Job drawing, mm, ordinate dimensions from the low corner. One solid piece. A direction names the side the tool comes from. Give positions to 0.01 mm unless a question says otherwise; leave off trailing zeros. Order: outer loops, then holes, each group sorted by start corner. A loop starts at its lowest first (then second) coordinate and runs counter-clockwise, first axis right, second up. Notation, with made-up numbers: M -1,75.5 L 12,75.5 A17 ccw 12,80.5 Z; hole C 48,87.5 d9. An arc over 180 degrees is marked long. Use CSV: the item, a comma, the result in double quotes. Start each with the question number.
Item 1: Band-saw the part on B-B on z = 31. Write the cut outline in (x, y).
Item 2: Band-saw the part on C-C on y = 132. Write the cut outline in (x, z).
Item 3: Wall check: line 1 along Z through (x, y) = (9, 16.25); line 2 along Y through (x, z) = (26, 17); line 3 along X through (y, z) = (132.5, 51). Give the ranges that are in metal, low to high.
Item 4: Pin check, flat tips, straight feed: P1, Ø6, axis at x = 108, y = 113, coming from the +Z side; P2, Ø9, axis at x = 6.5, y = 79, coming from the +Z side; P3, Ø4, axis at x = 21, y = 108, coming from the +Z side. Stop position of each tip, or through.
Item 5: Which spindle directions (+Z, -Z, +X, -X, +Y, -Y) get a long thin tool onto all of the face, cutting with end or side? Do the marked faces 1, 2 and 3. Say none if no direction does.
Item 6: Band-saw the part on A-A on x = 45.5. Write the cut outline in (y, z), plus the area to 3 significant figures.
Item 7: Band-saw the part on D-D on x = 9. Write the cut outline in (y, z).
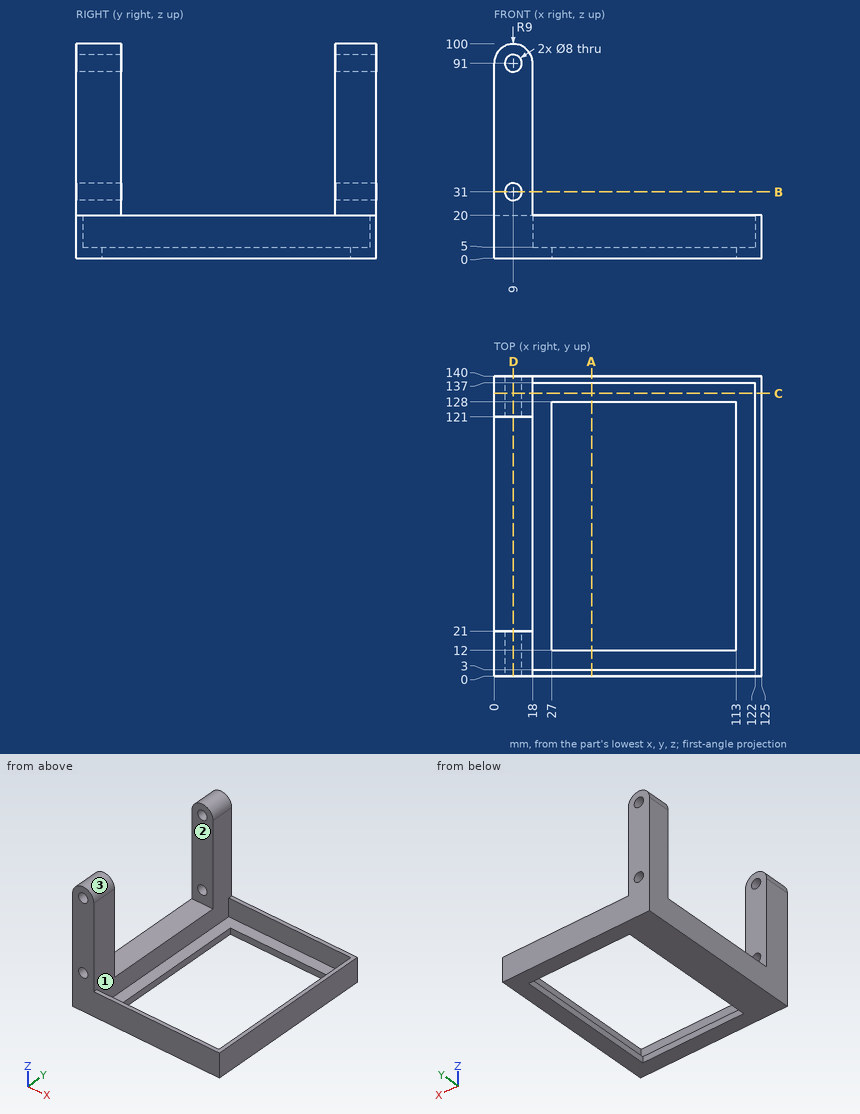
Model answer:
1,outline,"M 0,0 L 5,0 L 5,21 L 0,21 Z; M 0,121 L 5,121 L 5,140 L 0,140 Z; M 13,0 L 18,0 L 18,21 L 13,21 Z; M 13,121 L 18,121 L 18,140 L 13,140 Z"
2,outline,"M 0,0 L 125,0 L 125,20 L 122,20 L 122,5 L 18,5 L 18,91 A9 ccw 0,91 Z; hole C 9,31 d8; hole C 9,91 d8"
3,line 1,"z = 0 to 27, 35 to 87, 95 to 100"
3,line 2,"y = 0 to 3, 137 to 140"
3,line 3,"x = 0 to 18"
4,P1,"passes through"
4,P2,"stops at z = 20"
4,P3,"stops at z = 5"
5,face 1,"+Z"
5,face 2,"+Z, +X, -X"
5,face 3,"+Z, +Y, -Y"
6,outline,"M 0,0 L 12,0 L 12,5 L 3,5 L 3,20 L 0,20 Z; M 128,0 L 140,0 L 140,20 L 137,20 L 137,5 L 128,5 Z"
6,area,"210 mm^2"
7,outline,"M 0,0 L 140,0 L 140,27 L 121,27 L 121,20 L 21,20 L 21,27 L 0,27 Z; M 0,35 L 21,35 L 21,87 L 0,87 Z; M 0,95 L 21,95 L 21,100 L 0,100 Z; M 121,35 L 140,35 L 140,87 L 121,87 Z; M 121,95 L 140,95 L 140,100 L 121,100 Z"
